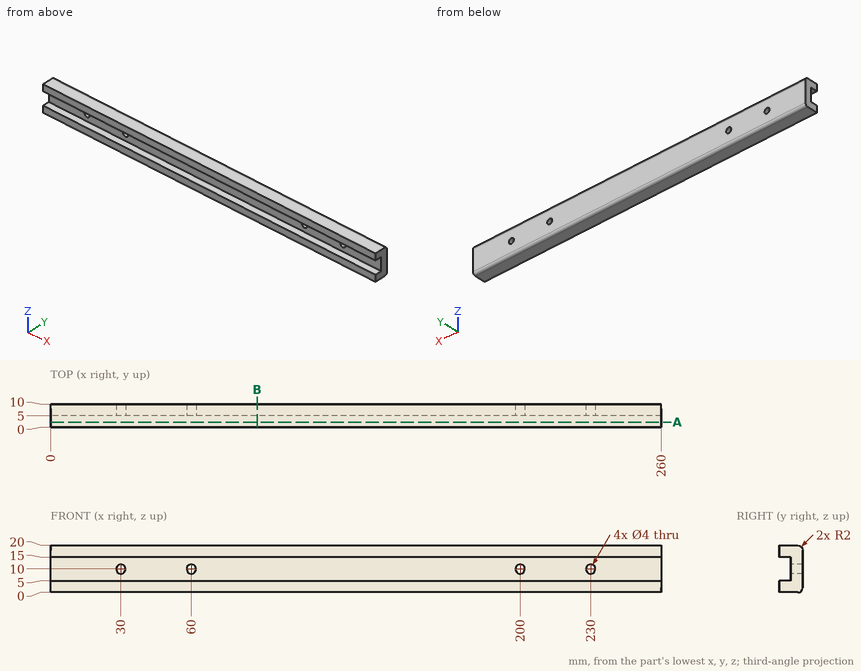
Geometry check sheet. Reference: drawing and pictorial views, mm from the part's lowest x, y, z. Give positions to 0.01 mm unless a question says otherwise; leave off trailing zeros. Loops run counter-clockwise (first coordinate to the right, second up) from the corner with the lowest first, then second, coordinate; pieces in that order, holes last. Notation, with made-up numbers: (12, -32) - (59, -32) arc R29 ccw to (59, 6) - close; hole circle Ø11 at (21.25, 40). An arc over 180 degrees is marked (long way). Use CSV: the item, a comma, the result in double quotes. Start each with the question number.
Q1. Scan lines: probe 1 along X at (y, z) = (6.35, 10); probe 2 along Z at (x, y) = (194, 3.5); probe 3 along Z at (x, y) = (30, 6.6). Record each from-to range of solid material in increasing order. Write a range as from..to.
Q2. Section check A-A, the plane y = 2.25. Record the cut outline in (x, z).
Q3. Section check B-B, the plane x = 88. Record the cut outline in (y, z).
Q4. Go/stop test with a flat-tipped pin: pin 1 Ø5 at (x, z) = (30, 10) entering from -Y. Record where the tip stops, or that it passes through.
Findings below:
1,probe 1,"x = 0..28, 32..58, 62..198, 202..228, 232..260"
1,probe 2,"z = 0..5, 15..20"
1,probe 3,"z = 0..8, 12..20"
2,outline,"(0, 0) - (260, 0) - (260, 5) - (0, 5) - close; (0, 15) - (260, 15) - (260, 20) - (0, 20) - close"
3,outline,"(0, 0) - (8, 0) arc R2 ccw to (10, 2) - (10, 18) arc R2 ccw to (8, 20) - (0, 20) - (0, 15) - (5, 15) - (5, 5) - (0, 5) - close"
4,pin 1,"stops at y = 5"
